Geometry: see drawing. Coordinates: mm, zero at the bounding-box minimum. A direction names the side the tool comes from. Coordinates: 2 decimals unless noted, no trailing zeros. Order: outer loops, then holes, each group sorted by start corner. A loop starts at its lowest first (then second) coordinate and runs counter-clockwise, first axis right, second up.
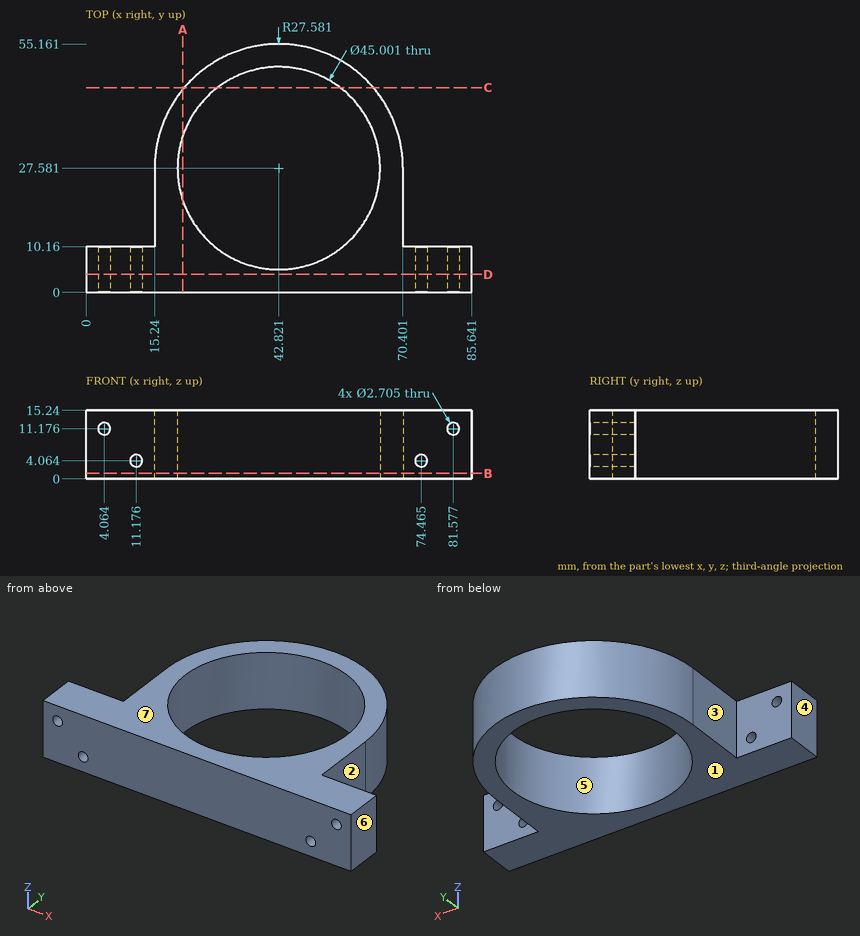
Item 1: Cut plane D-D on y = 4. Return loops of the section in (x, z) (1 decimal), then the cut area to 3 significant figures.
Response values:
outline: (0, 0) - (85.6, 0) - (85.6, 15.2) - (0, 15.2) - close; hole circle Ø2.7 at (4.1, 11.2); hole circle Ø2.7 at (11.2, 4.1); hole circle Ø2.7 at (74.5, 4.1); hole circle Ø2.7 at (81.6, 11.2)
area: 1,280 mm2
Item 2: Cut plane C-C on y = 45.5. Return loops of the section in (x, z) (1 decimal).
Response values:
outline: (21.9, 0) - (29.2, 0) - (29.2, 15.2) - (21.9, 15.2) - close; (56.4, 0) - (63.8, 0) - (63.8, 15.2) - (56.4, 15.2) - close
Item 3: Cut plane B-B on z = 1.25. Return loops of the section in (x, y).
Response values:
outline: (0, 0) - (85.64, 0) - (85.64, 10.16) - (70.4, 10.16) - (70.4, 27.58) arc R27.58 ccw to (15.24, 27.58) - (15.24, 10.16) - (0, 10.16) - close; hole circle Ø45 at (42.82, 27.58)
Item 4: Cut plane A-A on x = 21.5. Return loops of the section in (y, z).
Response values:
outline: (0, 0) - (20.39, 0) - (20.39, 15.24) - (0, 15.24) - close; (34.77, 0) - (45.08, 0) - (45.08, 15.24) - (34.77, 15.24) - close
Item 5: Access query for the marked faces 1, 2 and 3. Directions: +Z, -Z, +X, -X, +Y, -Y. A direction counts if a zero-diameter tool reaches every point of the face in a straight line with its end or side. Return the directions, or none.
Response values:
face 1: -Z, +X, -X, +Y, -Y
face 2: +Z, -Z, +X, +Y
face 3: +Z, -Z, -X, +Y
Item 6: Ray query, probe 1 along X at (y, z) = (27.5, 12.5); probe 2 along Y at (x, z) = (72, 13.25); probe 3 along X at (y, z) = (17, 10.25). Return the intervals inside material, ascending.
Response values:
probe 1: x = 15.24 to 20.32, 65.32 to 70.4
probe 2: y = 0 to 10.16
probe 3: x = 15.24 to 22.96, 62.68 to 70.4
Item 7: Draft query along X for the marked faces 4, 5, 6 and 7. Return one class per face: pulls with the +X half, pulls with the -X half, needs draft (parallel to the pull), parting line crosses it, or undercut.
Response values:
face 4: pulls with the -X half
face 5: undercut
face 6: pulls with the +X half
face 7: needs draft
Item 8: Pin query (flat end, axial travel): pin 1 Ø1 at (y, z) = (46, 5) entering from +X; pin 2 Ø4.5 at (x, z) = (4.5, 10) entering from +Y; pin 3 Ø2.5 at (x, z) = (74.47, 4.06) entering from +Y; pin 4 Ø7.5 at (y, z) = (17, 6) entering from +X. Return the tip coordinate at first contact, or that it passes through.
Response values:
pin 1: stops at x = 63.79
pin 2: stops at y = 10.16
pin 3: passes through
pin 4: stops at x = 70.4
